Check sheet for the modelled part. Datum: model origin and axes. Units: mm. A direction names the side the tool comes from. Coordinates: 2 decimals unless noted, no trailing zeros. Order: outer loops, then holes, each group sorted by start corner. A loop starts at its lowest first (then second) coordinate and runs counter-clockwise, first axis right, second up.
from build123d import *

# Parameters (mm, degrees)
SKETCH1_W           = 20
SKETCH1_H           = 60
SKETCH1_R           = 2.25
BOSS_EXTRUDE1_DEPTH = 5
SKETCH2_R           = 2.25
BOSS_EXTRUDE2_DEPTH = 10
SKETCH3_R           = 2.25
BOSS_EXTRUDE3_DEPTH = 10
CUT_EXTRUDE1_DEPTH  = 61


with BuildPart() as part:
    # Sketch1 → Boss-Extrude1 (new body)
    with BuildSketch(Plane(origin=(0, 0, 0), x_dir=(1, 0, 0), z_dir=(0, 1, 0))):
        Rectangle(SKETCH1_W, SKETCH1_H)
        with Locations((0, 25)):
            Circle(SKETCH1_R, mode=Mode.SUBTRACT)
        with Locations((0, -25)):
            Circle(SKETCH1_R, mode=Mode.SUBTRACT)
    extrude(amount=BOSS_EXTRUDE1_DEPTH)

    # Sketch2 → Boss-Extrude2 (add)
    with BuildSketch(Plane.XY.offset(20)):
        with BuildLine():
            Line((10, 9.86530346), (10, 5))
            Line((10, 5), (-6, 5))
            Line((-6, 5), (5.255684086, 19.53837663))
            ThreePointArc((5.255684086, 19.53837663), (15.386948998, 18.507420129), (10, 9.86530346))
        make_face()
        with Locations((10, 15.86530346)):
            Circle(SKETCH2_R, mode=Mode.SUBTRACT)
    extrude(amount=-BOSS_EXTRUDE2_DEPTH)

    # Sketch3 → Boss-Extrude3 (add)
    with BuildSketch(Plane(origin=(0, 0, -10), x_dir=(-1, 0, 0), z_dir=(0, 0, -1))):
        with BuildLine():
            Line((-10, 9.86530346), (-10, 5))
            Line((-10, 5), (6, 5))
            Line((6, 5), (-5.293415142, 19.586601483))
            ThreePointArc((-5.293415142, 19.586601483), (-15.40036055, 18.479898253), (-10, 9.86530346))
        make_face()
        with Locations((-10, 15.86530346)):
            Circle(SKETCH3_R, mode=Mode.SUBTRACT)
    extrude(amount=-BOSS_EXTRUDE3_DEPTH)

    # Sketch5 → Cut-Extrude1 (cut, through all)
    with BuildSketch(Plane(origin=(0, 0, -30), x_dir=(-1, 0, 0), z_dir=(0, 0, -1))):
        Polygon((-10, 9.86530346), (-10, 0), (-8.5, 0), align=None)
    extrude(amount=-CUT_EXTRUDE1_DEPTH, mode=Mode.SUBTRACT)


solid = part.part
(1) Tool access check on faces 1 (the flat face through (-7, 5, -7)), 2 (the flat face through (8, 14, 20)), 3 (the flat face through (8, 14, 10)). Record the directions out of +Z, -Z, +X, -X, +Y, -Y that give a thin tool (end or side, any length) a straight path to the whole face; none if there is none.
Filled in:
face 1: -X, +Y
face 2: +Z, +X, -X, +Y
face 3: +X, -X, +Y
(2) Cross-section at D-D (x = 0). Enter the section's corners in (y, z), and give its area (3 significant figures).
Filled in:
outline: (0, -30) - (5, -30) - (5, -27.25) - (0, -27.25) - close; (0, -22.75) - (5, -22.75) - (5, -10) - (12.75, -10) - (12.75, 0) - (5, 0) - (5, 10) - (12.75, 10) - (12.75, 20) - (5, 20) - (5, 22.75) - (0, 22.75) - close; (0, 27.25) - (5, 27.25) - (5, 30) - (0, 30) - close
area: 410 mm2
(3) Cross-section at A-A (z = 25). Enter the section's corners in (x, y), and give its area (3 significant figures).
Filled in:
outline: (-10, 0) - (-2.25, 0) - (-2.25, 5) - (-10, 5) - close; (2.25, 0) - (8.5, 0) - (9.26, 5) - (2.25, 5) - close
area: 71.9 mm2
(4) Cross-section at B-B (x = 11.25). Enter the section's corners in (y, z), and give its area (3 significant figures).
Filled in:
outline: (10, -10) - (13.99, -10) - (13.99, 0) - (10, 0) - close; (10, 10) - (13.99, 10) - (13.99, 20) - (10, 20) - close; (17.74, -10) - (21.73, -10) - (21.73, 0) - (17.74, 0) - close; (17.74, 10) - (21.73, 10) - (21.73, 20) - (17.74, 20) - close
area: 160 mm2
(5) Thickness scan on probe 1 along Z at (x, y) = (0, 3.2); probe 2 along Z at (x, y) = (3, 16.5); probe 3 along Y at (x, z) = (-7.25, -10.5). Record the ranges inside material, lowest first.
Filled in:
probe 1: z = -30 to -27.25, -22.75 to 22.75, 27.25 to 30
probe 2: z = -10 to 0, 10 to 20
probe 3: y = 0 to 5
(6) Release check for a two-part mould opening along X. For faces 4 (the cylindrical face through (9.707, 18.096, 15.07)), 5 (the cylindrical face through (10.293, 18.096, -5.07)), 6 (the flat face through (-0.432, 12.191, -5.07)), 7 (the flat face through (-1, 2, 30)) record: +X half, -X half, draft (parallel to the pull), parting line (faces both ways), or undercut.
Filled in:
face 4: undercut
face 5: undercut
face 6: -X half
face 7: draft
(7) Go/stop test with flat-tipped pins: P1, Ø6, axis at x = -3, y = 13.5, coming from the -Z side; P2, Ø8.5, axis at x = 0, y = 15.5, coming from the +Z side; P3, Ø3.5, axis at x = 0, z = 25, coming from the -Y side; P4, Ø9.5, axis at x = 3.5, z = -9, coming from the +Y side. Record where each tip stops, or that it passes through.
Filled in:
P1: stops at z = -10
P2: stops at z = 20
P3: passes through
P4: stops at y = 21.6
(8) Cross-section at C-C (y = 10.75). Enter the section's corners in (x, z), and give its area (3 significant figures).
Filled in:
outline: (-1.55, -10) - (13.14, -10) - (13.14, 0) - (-1.55, 0) - close; (-1.55, 10) - (13.14, 10) - (13.14, 20) - (-1.55, 20) - close
area: 294 mm2
